The figure shows three views and two pictorial views of one solid part (mm, origin at its lowest corner). Answer the questions. A direction names the side the tool comes from. Coordinates: 2 decimals unless noted, no trailing zeros. Loops run counter-clockwise (first coordinate to the right, second up) from the corner with the lowest first, then second, coordinate; pieces in that order, holes last. Notation, with made-up numbers: (-7, 54) - (47, 54) arc R12 ccw to (47, 75) - close; hole circle Ø8 at (-39.75, 60). An arc over 180 degrees is marked (long way). Write each question's results on one line, items separated by ' | '. Start each with the question number.
Item 1: Consider probe 1 along Z at (x, y) = (4, 4.75); probe 2 along Z at (x, y) = (3.75, 0.75); probe 3 along Z at (x, y) = (7, 4.75). Determine where each line is inside the solid, lowest interval first. Write a range as [from, to].
Item 2: A tool of negligible diameter and unlimited length cuts with its end or side. For the marked faces 4 and 5, from which of +Z, -Z, +X, -X, +Y, -Y can it reach the whole face along a straight path? Write none if from no direction.
Item 3: Each of these flat-tipped pins is pushed along its axis until it touches: pin 1 Ø1.5 at (y, z) = (1, 15) entering from +X; pin 2 Ø3.5 at (x, z) = (4, 16.55) entering from -Y (3 decimals). Where does it stop, or does it pass through?
Item 4: Section D-D, the plane x = 6 is taken. Write down the section's boundary in (y, z), plus the area to 3 significant figures.
Item 5: For a pull along Z with two mould halves and no side action, classify the marked faces 1, 2 and 3 as +Z half, -Z half, draft (parallel to the pull), parting line (faces both ways), or undercut.
Item 6: Section B-B, the plane y = 6 is taken. Write down the section's boundary in (x, z), plus the area to 3 significant figures.
Item 7: Section C-C, the plane z = 9.75 is taken. Write down the section's boundary in (x, y).
Item 8: Section A-A, the plane x = 4 is taken. Write down the section's boundary in (y, z) (3 decimals), plus the area to 3 significant figures.
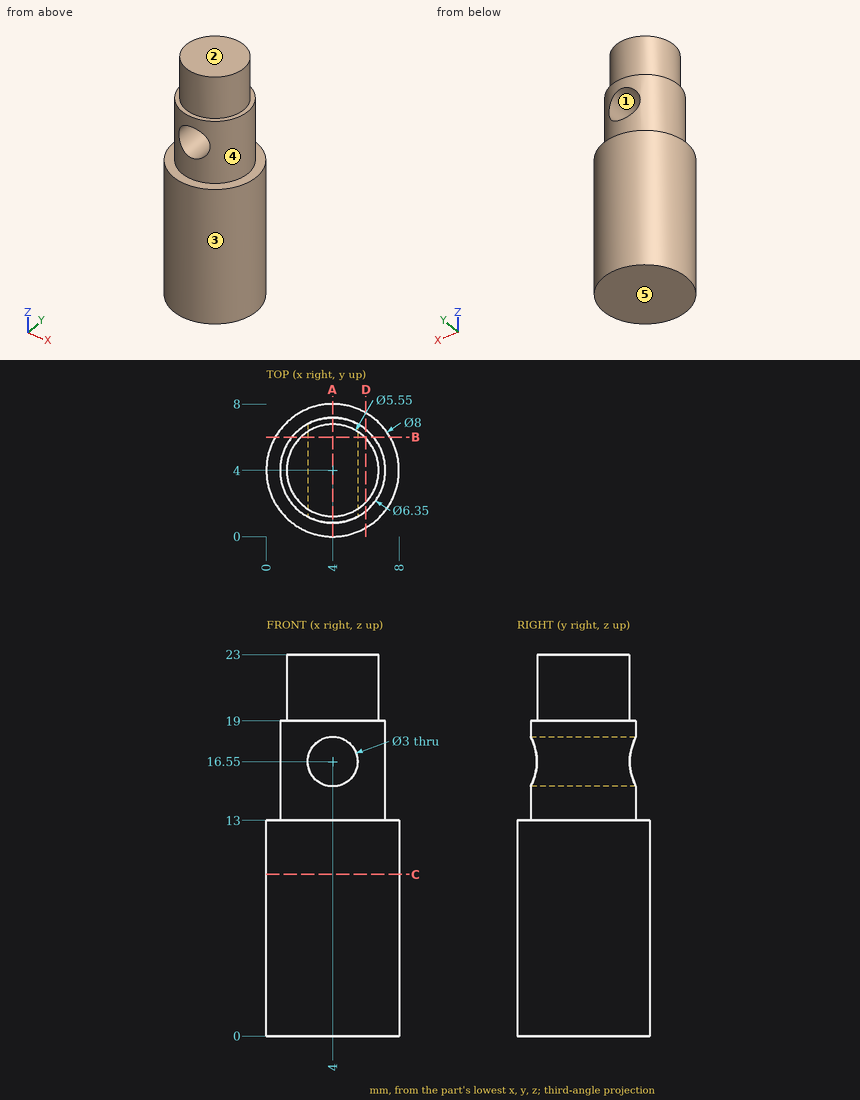
Answer key:
1) probe 1: z = [0, 15.05], [18.05, 23] | probe 2: z = [0, 13] | probe 3: z = [0, 19]
2) face 4: +Z | face 5: -Z, +X, -X, +Y, -Y
3) pin 1: stops at x = 6.24 | pin 2: stops at y = 0.825
4) outline: (0.54, 0) - (7.46, 0) - (7.46, 13) - (6.47, 13) - (6.47, 19) - (5.92, 19) - (5.92, 23) - (2.08, 23) - (2.08, 19) - (1.53, 19) - (1.53, 13) - (0.54, 13) - close | area: 135 mm^2
5) face 1: undercut | face 2: +Z half | face 3: draft
6) outline: (0.54, 0) - (7.46, 0) - (7.46, 13) - (6.47, 13) - (6.47, 19) - (5.92, 19) - (5.92, 23) - (2.08, 23) - (2.08, 19) - (1.53, 19) - (1.53, 13) - (0.54, 13) - close; hole circle Ø3 at (4, 16.55) | area: 128 mm^2
7) outline: circle Ø8 at (4, 4)
8) outline: (0, 0) - (8, 0) - (8, 13) - (7.175, 13) - (7.175, 15.05) - (0.825, 15.05) - (0.825, 13) - (0, 13) - close; (0.825, 18.05) - (7.175, 18.05) - (7.175, 19) - (6.775, 19) - (6.775, 23) - (1.225, 23) - (1.225, 19) - (0.825, 19) - close | area: 145 mm^2
